Autodesk Inventor part; units mm, degrees
ref_plane "YZ Plane" through (0, 0, 0) normal (1, 0, 0) x (0, 1, 0)
ref_plane "XZ Plane" through (0, 0, 0) normal (0, 1, 0) x (-1, 0, 0)
ref_plane "XY Plane" through (0, 0, 0) normal (0, 0, 1) x (1, 0, 0)
sketch "Sketch1" plane through (0, 0, 0) normal (1, 0, 0) x (0, 1, 0)
  line L0 (-13.5, 12.925) -> (13.5, 12.925)
  line L1 (13.5, 12.925) -> (13.5, -12.925)
  line L2 (13.5, -12.925) -> (-13.5, -12.925)
  line L3 (-13.5, -12.925) -> (-13.5, 12.925)
  line L4 (-13.5, 12.925) -> (13.5, -12.925) construction
  line L5 (13.5, 12.925) -> (-13.5, -12.925) construction
  circle A0 centre (-7.65, -7.075) radius 8 construction
  line L6 (-5.5, 12.925) -> (-5.5, 10.887)
  circle A1 centre (-7.65, -7.075) radius 2.75
  line L7 (-1.8, -12.925) -> (-1.8, -2.075)
  arc A2 (3.2, 2.925) -> (-1.8, -2.075) centre (3.2, -2.075) ccw
  line L8 (3.2, 2.925) -> (13.5, 2.925)
  point P0 (0, 0)
  dimension "d0" = 27
  dimension "d1" = 25.85
  dimension "d2" = 16
  dimension "d3" = 21.15
  dimension "d4" = 19
  dimension "d5" = 20
  dimension "d6" = 5.5
  dimension "d7" = 5.85
  dimension "d8" = 5.85
  dimension "d9" = 5.85
  dimension "d10" = 10
  dimension "d11" = 5
extrude "Extrusion1" add sketch "Sketch1" along normal mid plane 15 contours L0 L1 L8 A2 L7 L2 L3
fillet "Fillet1" radius 5 3 edges at (0, -1.8, -12.925) (0, -13.5, -12.925) (0, 13.5, 2.925)
sketch "Sketch2" plane through (0, 0, 0) normal (1, 0, 0) x (0, 1, 0)
  arc A0 (8.5, 2.925) -> (13.5, 7.925) centre (8.5, 7.925) ccw
  line L0 (13.5, 7.925) -> (13.5, 12.925)
  line L1 (13.5, 12.925) -> (-13.5, 12.925)
  line L2 (-13.5, 12.925) -> (-13.5, -7.925)
  arc A1 (-13.5, -7.925) -> (-8.5, -12.925) centre (-8.5, -7.925) ccw
  line L3 (-8.5, -12.925) -> (-6.8, -12.925)
  arc A2 (-6.8, -12.925) -> (-1.8, -7.925) centre (-6.8, -7.925) ccw
  line L4 (-1.8, -7.925) -> (-1.8, -2.075)
  arc A3 (3.2, 2.925) -> (-1.8, -2.075) centre (3.2, -2.075) ccw
  line L5 (3.2, 2.925) -> (8.5, 2.925)
  circle A4 centre (-7.65, -7.075) radius 2.75
  circle A5 centre (-7.65, -7.075) radius 10
  point P0 (0, 0)
  dimension "d15" = 20
extrude "Extrusion2" cut sketch "Sketch2" against normal mid plane 7 contours A5 L2 A1 L3 A2 L4 A3 | A3 L4 A2 L3 A1 L2 A5 | A4
fillet "Fillet2" radius 5 2 edges at (0, -1.0981, 0.4797) (0, -13.5, 1.0353)
sketch "Sketch3" plane through (-7.5, -13.5, 12.925) normal (0, 0, 1) x (1, 0, 0)
  line L0 (0, 27) -> (15, 27)
  point P0 (7.5, 13.5)
  point P1 (7.5, 20)
  point P2 (7.5, 8)
  dimension "d19" = 7
  dimension "d20" = 19
hole "Hole1" at (0, 6.5, 12.925) at (0, -5.5, 12.925) direction (0, 0, -1) diameter 7.8 depth 6.7 countersink diameter 8.3 countersink angle 8
sketch "Sketch4" plane through (-7.5, -13.5, 12.925) normal (0, 0, 1) x (1, 0, 0)
  circle A0 centre (7.5, 20) radius 3.9
  circle A1 centre (7.5, 8) radius 3.9
  point P0 (7.5, 13.5)
hole "Hole2" at (0, 6.5, 12.925) at (0, -5.5, 12.925) direction (0, 0, -1) diameter 5.5 end through all
fillet "Fillet3" radius 2 18 edges at (7.5, 5.85, 2.925) (7.5, -0.3355, 1.4605) (7.5, -1.8, -5) (7.5, -3.2645, -11.4605) (7.5, -7.65, -12.925) (7.5, -12.0355, -11.4605) (7.5, -13.5, 2.5) (7.5, 13.5, 10.425) (7.5, 12.0355, 4.3895) (-7.5, 13.5, 10.425) (-7.5, 5.85, 2.925) (-7.5, -0.3355, 1.4605) (-7.5, -1.8, -5) (-7.5, -3.2645, -11.4605) (-7.5, -7.65, -12.925) (-7.5, -12.0355, -11.4605) (-7.5, -13.5, 2.5) (-7.5, 12.0355, 4.3895)
equation "\"d8\" = d7"
equation "\"d9\" = d7"
properties part number "Y-Axis_Belt_Bearing_Mount_LM3045" material "ABS Plastic"
Work out the finished part from the listing and answer in its coordinate system (mm). A direction names the side the tool comes from. Round coordinates to 2 decimals unless told otherwise and drop trailing zeros. Loops run counter-clockwise (first coordinate to the right, second up) from the corner with the lowest first, then second, coordinate; pieces in that order, holes last. Notation, with made-up numbers: M -22.5,38 L -5.5,38 A21 ccw -5.5,45 Z; hole C -8.75,-16.5 d9. An arc over 180 degrees is marked long. Use CSV: the item, a comma, the result in double quotes.
Q1. A tool of negligible diameter and unlimited length cuts with its end or side. For faces 1 (the cylindrical face through (2.97, -6.43, 2.85)), 2 (the flat face through (-3.5, -8, -2)), 3 (the cylindrical face through (6.93, 5.887, 3.526)), 4 (the flat face through (4, -1.8, -5)), 5 (the cylindrical face through (-1.17, 2.78, 7.77)), from which of +Z, -Z, +X, -X, +Y, -Y can it reach the whole face along a straight path? Write none if from no direction.
Determined:
face 1,"-Z"
face 2,"-Z, -Y"
face 3,"-Z, +X, +Y"
face 4,"-Z, +X, -X, +Y"
face 5,"+Z"
Q2. Section C-C, the plane z = -3 is taken. Determine the outline of the cut face in (x, y), then the cut area to 3 significant figures.
Determined:
outline,"M -7.5,-11.5 A2 ccw -5.5,-13.5 L -3.5,-13.5 L -3.5,-1.8 L -5.5,-1.8 A2 ccw -7.5,-3.8 Z; M 3.5,-13.5 L 5.5,-13.5 A2 ccw 7.5,-11.5 L 7.5,-3.8 A2 ccw 5.5,-1.8 L 3.5,-1.8 Z"
area,"90.2 mm2"
Q3. Each of these flat-tipped pins is pushed along its axis until it touches: pin 1 (4 mm diameter, centred on x = 6, z = -4, fed in from +Y); pin 2 (2.5 mm diameter, centred on x = -0.5, y = 8, fed in from +Z) (3 decimals); pin 3 (1.5 mm diameter, centred on x = 3.5, y = 8.5, fed in from -Z) (3 decimals). Where does it stop, or does it pass through?
Determined:
pin 1,"y = -1.8"
pin 2,"z = 6.225"
pin 3,"z = 2.925"
Q4. Section D-D, the plane x = 0 is taken. State how many separate pieces and enclosed holes the cut face has, then the cut area to 3 significant figures.
Determined:
separate pieces,"3"
enclosed holes,"0"
area,"121 mm2"
Q5. The mould has two halves that part along Z. Classify faces 6 (the cylindrical face through (5.47, -9.68, -8.93)), 7 (the conical face through (1.201, -9.314, 10.765)), 8 (the cylindrical face through (-3.01, -6.43, 2.85)): pulls with the +Z half, pulls with the -Z half, needs draft (parallel to the pull), parting line crosses it, or undercut.
Determined:
face 6,"undercut"
face 7,"pulls with the +Z half"
face 8,"pulls with the -Z half"
Q6. Section B-B, the plane y = 6.5 is taken. Determine the outline of the cut face in (x, z) (3 decimals).
Determined:
outline,"M -7.5,4.925 A2 ccw -5.5,2.925 L -2.75,2.925 L -2.75,6.225 L -3.9,6.225 L -3.9,9.35 L -4.15,12.925 L -7.5,12.925 Z; M 2.75,2.925 L 5.5,2.925 A2 ccw 7.5,4.925 L 7.5,12.925 L 4.15,12.925 L 3.9,9.35 L 3.9,6.225 L 2.75,6.225 Z"
Q7. Consider L1, parallel to Y at x = 0, z = 8; L2, parallel to Y at x = 0, z = 5.1; L3, parallel to X at y = -10.5, z = -2.25. Determine where each line is inside the solid, lowest interval first.
Determined:
L1,"-13.5 to -9.4, -1.6 to 2.6, 10.4 to 13.5"
L2,"-12.64 to -8.25, -2.75 to 3.75, 9.25 to 12.63"
L3,"-7.5 to -3.5, 3.5 to 7.5"
Q8. Section A-A, the plane z = 8.5 is taken. Determine the outline of the cut face in (x, y).
Determined:
outline,"M -7.5,-11.5 A2 ccw -5.5,-13.5 L 5.5,-13.5 A2 ccw 7.5,-11.5 L 7.5,11.5 A2 ccw 5.5,13.5 L -5.5,13.5 A2 ccw -7.5,11.5 Z; hole C 0,-5.5 d7.8; hole C 0,6.5 d7.8"
